Build history of the part. All positions in model axes, mm. Face numbers are marked on the shaded views. A direction names the side the tool comes from. Round coordinates to 2 decimals unless told otherwise and drop trailing zeros. Write each loop counter-clockwise with the first axis right and the second up, starting at its lowest first coordinate (ties: lowest second). Pieces come first, ordered by that corner, then holes. Notation, with made-up numbers: M 19,-12 L 63,-12 A23 ccw 63,4 Z; hole C 49.5,64 d10. An arc over 180 degrees is marked long. Use a Markdown table: item, result.
Autodesk Inventor part; units mm, degrees
ref_plane "Work Plane1" through (-31.75, -10.525, -6.35) normal (0, 0, -1) x (0, 1, 0)
ref_plane "YZ Plane" through (0, 0, 0) normal (1, 0, 0) x (0, 1, 0)
ref_plane "XZ Plane" through (0, 0, 0) normal (0, 1, 0) x (-1, 0, 0)
sketch "Sketch1" plane through (0, 0, 0) normal (0, 0, 1) x (1, 0, 0)
  line L0 (-22.235, -36.3697) -> (-22.235, -26.7755)
  line L1 (-22.235, -26.7755) -> (-25.9663, -26.7755)
  line L2 (-26.045, -26.8374) -> (-26.045, -30.1399)
  arc A0 (-26.045, -30.1399) -> (-26.045, -34.0927) centre (-24.7167, -32.1163) ccw
  line L3 (-26.045, -34.0927) -> (-26.045, -36.3697)
  line L4 (-26.045, -36.3697) -> (-31.75, -36.3697)
  line L5 (-31.75, -36.3697) -> (-31.75, -19.7975)
  line L6 (-31.75, -19.7975) -> (31.75, -19.7975)
  line L7 (31.75, -19.7975) -> (31.75, -36.3697)
  line L8 (31.75, -36.3697) -> (-22.235, -36.3697)
  line L9 (24.7167, -22.9725) -> (-19.6375, -22.9725)
  arc A1 (-19.6375, -22.9725) -> (-19.6375, -28.1475) centre (-19.6375, -25.56) ccw
  line L10 (-19.6375, -28.1475) -> (24.7167, -28.1475)
  arc A2 (24.7167, -28.1475) -> (24.7167, -22.9725) centre (24.7167, -25.56) ccw
  line L11 (-18.6822, -29.735) -> (-18.6822, -34.4975)
  line L12 (-18.6822, -34.4975) -> (24.7167, -34.4975)
  arc A3 (24.7167, -34.4975) -> (24.7167, -29.735) centre (24.7167, -32.1163) ccw
  line L13 (24.7167, -29.735) -> (-18.6822, -29.735)
  line L14 (-31.75, 25.8027) -> (31.75, 25.8027)
  line L15 (31.75, 25.8027) -> (31.75, 15.6277)
  line L16 (31.75, 15.6277) -> (-31.75, 15.6277)
  line L17 (-31.75, 15.6277) -> (-31.75, 25.8027)
  circle A4 centre (-26.9875, 20.7152) radius 1.5875
  line L18 (-26.9875, 20.7152) -> (-26.9875, 4.175)
  line L19 (-19.4952, 20.7152) -> (24.859, 20.7152) construction
  line L20 (-19.4952, 18.1277) -> (24.859, 18.1277)
  line L21 (24.859, 23.3027) -> (-19.4952, 23.3027)
  arc A5 (-19.4952, 23.3027) -> (-19.4952, 18.1277) centre (-19.4952, 20.7152) ccw
  arc A6 (24.859, 18.1277) -> (24.859, 23.3027) centre (24.859, 20.7152) ccw
  line L22 (12.1015, 23.3027) -> (12.1015, 18.1277) construction
  line L23 (12.1015, -22.9725) -> (12.1015, -28.1475) construction
  line L24 (-31.75, 20.7152) -> (-23.8125, 20.7152) construction
  arc A7 (-25.9663, -26.7755) -> (-26.045, -26.8374) centre (-26.9875, -25.56) ccw
  point P0 (0, 0)
  point P1 (2.6819, 20.7152)
  dimension "d0" = 2.5
  dimension "d5" = 44.3542
ref_plane "Work Plane1" through (-31.75, -10.525, -6.35) normal (0, 0, -1) x (0, 1, 0)
extrude "Extrusion1" add sketch "Sketch1" against normal up to surface (6.35 mm away) contours L14 L15 L16 L17
sketch "Sketch2" plane through (31.75, 15.6277, -6.35) normal (0, 0, -1) x (-1, 0, 0)
  point P0 (31.75, -15.6277)
sketch "Sketch3" plane through (-31.75, 25.8027, 0) normal (0, 1, 0) x (1, 0, 0)
  line L0 (0.254, -20.066) -> (0.254, 30.48)
  arc A0 (6.604, 36.83) -> (0.254, 30.48) centre (6.604, 30.48) ccw
  line L1 (6.604, 36.83) -> (57.15, 36.83)
  arc A1 (63.5, 30.48) -> (57.15, 36.83) centre (57.15, 30.48) ccw
  line L2 (63.5, -20.066) -> (63.5, 30.48)
  arc A2 (57.15, -26.416) -> (63.5, -20.066) centre (57.15, -20.066) ccw
  line L3 (6.604, -26.416) -> (57.15, -26.416)
  arc A3 (0.254, -20.066) -> (6.604, -26.416) centre (6.604, -20.066) ccw
  circle A4 centre (59.817, 30.607) radius 1.4732
  circle A5 centre (3.937, 30.607) radius 1.4732
  circle A6 centre (59.817, -20.193) radius 1.4732
  circle A7 centre (3.937, -20.193) radius 1.4732
  line L4 (63.5, 0) -> (0, 0)
  line L5 (0, 0) -> (63.5, 0)
  line L6 (9.0714, 0) -> (22.6786, 0)
  line L7 (22.6786, 0) -> (22.6786, -7.9375)
  line L8 (22.6786, -7.9375) -> (9.0714, -7.9375)
  line L9 (9.0714, -7.9375) -> (9.0714, 0)
  line L10 (63.5, 6.35) -> (0, 6.35)
  line L11 (22.6786, 6.35) -> (9.0714, 6.35)
  line L12 (9.0714, 6.35) -> (9.0714, 12.7)
  line L13 (9.0714, 12.7) -> (22.6786, 12.7)
  line L14 (22.6786, 12.7) -> (22.6786, 6.35)
  line L15 (56.2674, 0) -> (42.6602, 0)
  line L16 (42.6602, 0) -> (42.6602, -7.9375)
  line L17 (42.6602, -7.9375) -> (56.2674, -7.9375)
  line L18 (56.2674, -7.9375) -> (56.2674, 0)
  line L19 (0, 6.35) -> (63.5, 6.35)
  line L20 (56.2674, 6.35) -> (42.6602, 6.35)
  line L21 (42.6602, 6.35) -> (42.6602, 14.2875)
  line L22 (42.6602, 14.2875) -> (56.2674, 14.2875)
  line L23 (56.2674, 14.2875) -> (56.2674, 6.35)
  point P0 (31.75, 0)
extrude "Extrusion2" add sketch "Sketch3" against normal blind 1.5875 contours L4 L7 L8 L9 | L12 L13 L14 L10 | L4 L18 L17 L16 | L21 L22 L23 L10
sketch "Sketch4" plane through (-31.75, 25.8027, 0) normal (0, 1, 0) x (1, 0, 0)
  line L0 (63.5, 6.35) -> (56.2674, 6.35)
  line L1 (56.2674, 6.35) -> (56.2674, 14.2875)
  line L2 (56.2674, 14.2875) -> (42.6602, 14.2875)
  line L3 (42.6602, 14.2875) -> (42.6602, 6.35)
  line L4 (42.6602, 6.35) -> (22.6786, 6.35)
  line L5 (22.6786, 6.35) -> (22.6786, 12.7)
  line L6 (22.6786, 12.7) -> (9.0714, 12.7)
  line L7 (9.0714, 12.7) -> (9.0714, 6.35)
  line L8 (9.0714, 6.35) -> (0, 6.35)
  line L9 (0, 0) -> (0, 6.35)
  line L10 (9.0714, 0) -> (0, 0)
  line L11 (9.0714, 0) -> (9.0714, -7.9375)
  line L12 (9.0714, -7.9375) -> (22.6786, -7.9375)
  line L13 (22.6786, -7.9375) -> (22.6786, 0)
  line L14 (42.6602, 0) -> (22.6786, 0)
  line L15 (42.6602, 0) -> (42.6602, -7.9375)
  line L16 (42.6602, -7.9375) -> (56.2674, -7.9375)
  line L17 (56.2674, -7.9375) -> (56.2674, 0)
  line L18 (63.5, 0) -> (56.2674, 0)
  line L19 (63.5, 0) -> (63.5, 6.35)
  circle A0 centre (49.4638, -3.9688) radius 1.5
  circle A1 centre (49.4638, 10.3188) radius 1.5
  circle A2 centre (15.875, -3.9688) radius 1.5
  circle A3 centre (15.875, 9.525) radius 1.5
  point P0 (31.75, 0)
  dimension "d6" = 3
  dimension "d7" = 3
  dimension "d8" = 3
  dimension "d9" = 3
extrude "Extrusion3" cut sketch "Sketch4" against normal through all contours A0 | A1 | A2 | A3
properties part number "_3DPrint"
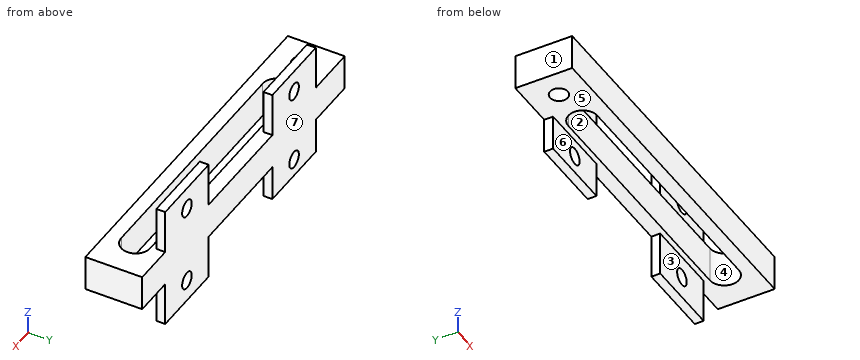
Q1. Drill centre lines: L1, parallel to X at y = 24.75, z = -9; L2, parallel to Y at x = 16.5, z = -0.5; L3, parallel to Z at x = -27, y = 22.5. Where is each one in solid material? Low to high.
Response values:
| item | result |
|---|---|
| L1 | x = -22.68 to -17.28, -14.47 to -9.07, 10.91 to 17, 18.43 to 24.52 |
| L2 | y = 15.63 to 18.13, 23.3 to 25.8 |
| L3 | z = -6.35 to 0 |
Q2. Cut at A-A on x = -12. Give the cut face in (y, z).
Response values:
| item | result |
|---|---|
| outline | M 15.63,-6.35 L 18.13,-6.35 L 18.13,0 L 15.63,0 Z; M 23.3,-6.35 L 24.22,-6.35 L 24.22,-12.7 L 25.8,-12.7 L 25.8,7.94 L 24.22,7.94 L 24.22,0 L 23.3,0 Z |
Q3. Two-plate mould, pull along Y, no slides. Class the marked faces 4, 5, 6 and 7: +Y half, -Y half, draft (parallel to the pull), parting line (faces both ways), or undercut.
Response values:
| item | result |
|---|---|
| face 4 | undercut |
| face 5 | draft |
| face 6 | -Y half |
| face 7 | +Y half |
Q4. Cut at C-C on y = 21.75. Give the cut face in (x, z).
Response values:
| item | result |
|---|---|
| outline | M -31.75,-6.35 L -28.19,-6.35 L -28.19,0 L -31.75,0 Z; M -25.78,-6.35 L -21.87,-6.35 L -21.87,0 L -25.78,0 Z; M 27.23,-6.35 L 31.75,-6.35 L 31.75,0 L 27.23,0 Z |
Q5. Cut at B-B on z = 1. Give the cut face in (x, y).
Response values:
| item | result |
|---|---|
| outline | M -22.68,24.22 L -9.07,24.22 L -9.07,25.8 L -22.68,25.8 Z; M 10.91,24.22 L 24.52,24.22 L 24.52,25.8 L 10.91,25.8 Z |
Q6. Which spindle directions (+Z, -Z, +X, -X, +Y, -Y) get a long thin tool onto all of the face, cutting with end or side? Do the marked faces 1, 2 and 3. Say none if no direction does.
Response values:
| item | result |
|---|---|
| face 1 | +Z, -Z, -X, +Y, -Y |
| face 2 | +Z, -Z |
| face 3 | -Z, +X, -X, -Y |
Q7. Cut at D-D on y = 25. Count the separate pieces of the cut face and the enclosed holes in it, and give its area (3 significant figures).
Response values:
| item | result |
|---|---|
| separate pieces | 1 |
| enclosed holes | 4 |
| area | 785 mm2 |
Q8. Drop flat-ended pins along their axis: P1, Ø8.5, axis at x = 19, z = -11, coming from the -Y side; P2, Ø4, axis at x = 21.5, y = 20, coming from the +Z side; P3, Ø1.3, axis at x = -19, y = 25, coming from the -Z side. Give the stop position or say it passes through.
Response values:
| item | result |
|---|---|
| P1 | stops at y = 24.22 |
| P2 | stops at z = 0 |
| P3 | stops at z = -12.7 |
